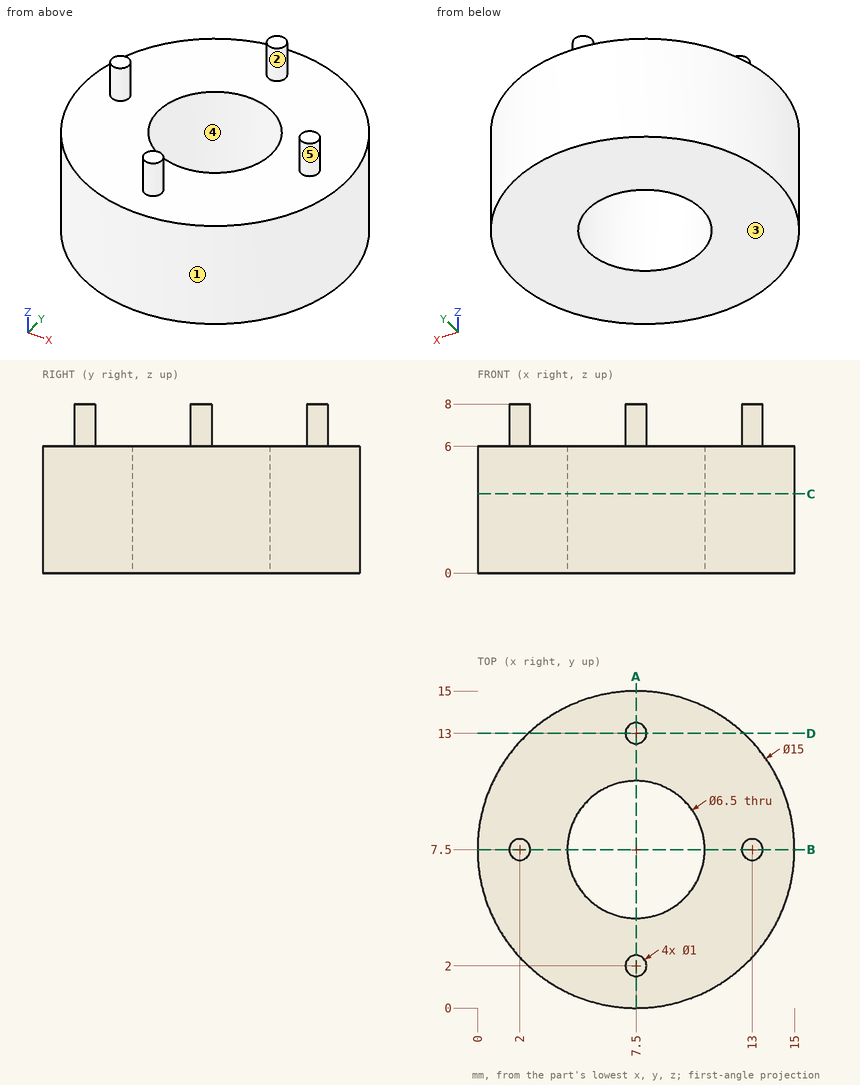
Verification items for this drawing (mm, ordinates from the low corner). A direction names the side the tool comes from. Coordinates: 2 decimals unless noted, no trailing zeros. Loops run counter-clockwise (first coordinate to the right, second up) from the corner with the lowest first, then second, coordinate; pieces in that order, holes last.
Item 1: Release check for a two-part mould opening along Y. For the marked faces 1, 2 and 3 record: released by +Y, released by -Y, zero draft, split by the parting line, or undercut.
Item 2: Thickness scan on line 1 (Y direction, x = 7.5, z = 3.7); line 2 (Z direction, x = 8, y = 12); line 3 (Y direction, x = 8.5, z = 5.75). Record the ranges inside material, lowest first.
Item 3: Sectioned sample at A-A, the plane x = 7.5. Record the boundary of the cut face in (y, z), then the cut area to 3 significant figures.
Item 4: Sectioned sample at C-C, the plane z = 3.75. Record the boundary of the cut face in (x, y).
Item 5: Sectioned sample at D-D, the plane y = 13. Record the boundary of the cut face in (x, z), then the cut area to 3 significant figures.
Item 6: Go/stop test with flat-tipped pins: pin 1 Ø4.5 at (x, y) = (6, 9.5) entering from +Z; pin 2 Ø1.5 at (x, z) = (12.5, 3.5) entering from +Y; pin 3 Ø1.5 at (y, z) = (13, 7) entering from -X; pin 4 Ø5 at (x, y) = (10.5, 5.5) entering from -Z. Record where each tip stops, or that it passes through.
Item 7: Access from +Z, -Z, +X, -X, +Y, -Y to the whole of each face (thin tool, end or side, straight path). Record for the marked faces 4 and 5.
Check result:
1. face 1: split by the parting line
1. face 2: undercut
1. face 3: zero draft
2. line 1: y = 0 to 4.25, 10.75 to 15
2. line 2: z = 0 to 6
2. line 3: y = 0.07 to 4.41, 10.59 to 14.93
3. outline: (0, 0) - (4.25, 0) - (4.25, 6) - (2.5, 6) - (2.5, 8) - (1.5, 8) - (1.5, 6) - (0, 6) - close; (10.75, 0) - (15, 0) - (15, 6) - (13.5, 6) - (13.5, 8) - (12.5, 8) - (12.5, 6) - (10.75, 6) - close
3. area: 55.0 mm2
4. outline: circle Ø15 at (7.5, 7.5); hole circle Ø6.5 at (7.5, 7.5)
5. outline: (2.4, 0) - (12.6, 0) - (12.6, 6) - (8, 6) - (8, 8) - (7, 8) - (7, 6) - (2.4, 6) - close
5. area: 63.2 mm2
6. pin 1: stops at z = 6
6. pin 2: stops at y = 13.68
6. pin 3: stops at x = 7
6. pin 4: stops at z = 0
7. face 4: +Z, -Z
7. face 5: +Z
